```python
from build123d import *

# Parameters (mm, degrees)
SKETCH_1_R          = 48.25
EXTRUDE_1_DEPTH     = 27.7
SKETCH_2_R          = 29
EXTRUDE_2_DEPTH     = 8
SKETCH_3_R          = 29.5
SKETCH_3_R_2        = 2
SKETCH_3_R_3        = 7.5
EXTRUDE_3_DEPTH     = 6.7
SKETCH_4_R          = 1.75
CUT_EXTRUDE_1_DEPTH = 5
SKETCH_5_R          = 1.75
CUT_EXTRUDE_2_DEPTH = 5
CUT_EXTRUDE_3_DEPTH = 36.7


with BuildPart() as part:
    # 草图1 → 凸台-拉伸1 (new body)
    with BuildSketch(Plane.XY):
        Circle(SKETCH_1_R)
    extrude(amount=EXTRUDE_1_DEPTH)

    # 草图2 → 凸台-拉伸2 (add)
    with BuildSketch(Plane(origin=(0, 0, 0), x_dir=(-1, 0, 0), z_dir=(0, 0, -1))):
        Circle(SKETCH_2_R)
    extrude(amount=EXTRUDE_2_DEPTH)

    # 草图3 → 凸台-拉伸3 (add)
    with BuildSketch(Plane.XY.offset(27.7)):
        Circle(SKETCH_3_R)
        with Locations((0, 17.25)):
            Circle(SKETCH_3_R_2, mode=Mode.SUBTRACT)
        with Locations((14.938938215, 8.625)):
            Circle(SKETCH_3_R_2, mode=Mode.SUBTRACT)
        with Locations((14.938938215, -8.625)):
            Circle(SKETCH_3_R_2, mode=Mode.SUBTRACT)
        with Locations((0, -17.25)):
            Circle(SKETCH_3_R_2, mode=Mode.SUBTRACT)
        with Locations((-14.938938215, -8.625)):
            Circle(SKETCH_3_R_2, mode=Mode.SUBTRACT)
        with Locations((-14.938938215, 8.625)):
            Circle(SKETCH_3_R_2, mode=Mode.SUBTRACT)
        Circle(SKETCH_3_R_3, mode=Mode.SUBTRACT)
    extrude(amount=EXTRUDE_3_DEPTH)

    # 草图4 → 切除-拉伸1 (cut)
    with BuildSketch(Plane.XY.offset(27.7)):
        with Locations((0, 44.5)):
            Circle(SKETCH_4_R)
        with Locations((31.466251763, 31.466251763)):
            Circle(SKETCH_4_R)
        with Locations((31.466251763, -31.466251763)):
            Circle(SKETCH_4_R)
        with Locations((0, -44.5)):
            Circle(SKETCH_4_R)
        with Locations((-31.466251763, -31.466251763)):
            Circle(SKETCH_4_R)
        with Locations((-31.466251763, 31.466251763)):
            Circle(SKETCH_4_R)
        with Locations((-42.5, 0)):
            Circle(SKETCH_4_R)
        with Locations((42.5, 0)):
            Circle(SKETCH_4_R)
    extrude(amount=-CUT_EXTRUDE_1_DEPTH, mode=Mode.SUBTRACT)

    # 草图5 → 切除-拉伸2 (cut)
    with BuildSketch(Plane(origin=(0, 0, 0), x_dir=(-1, 0, 0), z_dir=(0, 0, -1))):
        with Locations((0, 42.5)):
            Circle(SKETCH_5_R)
        with Locations((30.0520382, 30.0520382)):
            Circle(SKETCH_5_R)
        with Locations((42.5, 0)):
            Circle(SKETCH_5_R)
        with Locations((30.0520382, -30.0520382)):
            Circle(SKETCH_5_R)
        with Locations((0, -42.5)):
            Circle(SKETCH_5_R)
        with Locations((-30.0520382, -30.0520382)):
            Circle(SKETCH_5_R)
        with Locations((-42.5, 0)):
            Circle(SKETCH_5_R)
        with Locations((-30.0520382, 30.0520382)):
            Circle(SKETCH_5_R)
    extrude(amount=-CUT_EXTRUDE_2_DEPTH, mode=Mode.SUBTRACT)

    # 草图6 → 切除-拉伸3 (cut, through all)
    with BuildSketch(Plane.XY.offset(27.7)):
        with BuildLine():
            Line((-46.25, 13.747727085), (-46.25, -13.747727085))
            ThreePointArc((-46.25, -13.747727085), (-48.25, 0), (-46.25, 13.747727085))
        make_face()
        with BuildLine():
            Line((46.25, -13.747727085), (46.25, 13.747727085))
            ThreePointArc((46.25, 13.747727085), (48.25, 0), (46.25, -13.747727085))
        make_face()
    extrude(amount=-CUT_EXTRUDE_3_DEPTH, mode=Mode.SUBTRACT)


solid = part.part
```
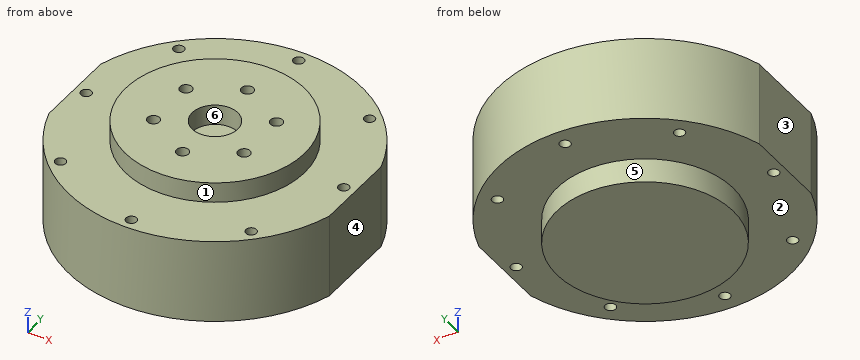
Here's how the part is built. I have some questions about the finished solid (model axes, mm). Face numbers are marked on the shaded views. A direction names the side the tool comes from. Round coordinates to 2 decimals unless told otherwise and drop trailing zeros. Loops run counter-clockwise (first coordinate to the right, second up) from the corner with the lowest first, then second, coordinate; pieces in that order, holes last.
1. Suppose I cut it at B-B, the plane x = -19.5. Please give me the cut outline in (y, z), and give its area (3 significant figures).
Answers:
outline: (-44.13, 0) - (-21.47, 0) - (-21.47, -8) - (21.47, -8) - (21.47, 0) - (44.13, 0) - (44.13, 27.7) - (22.14, 27.7) - (22.14, 34.4) - (-22.14, 34.4) - (-22.14, 27.7) - (-44.13, 27.7) - close
area: 3,090 mm2
2. For the marked faces 1, 2 and 3, which set-ups out of +Z, -Z, +X, -X, +Y, -Y let a thin tool reach every point of the face, with its end or its side?
Answers:
face 1: +Z
face 2: -Z
face 3: +Z, -Z, -X, +Y, -Y
3. Will these pins go through, and if not, where does the flat tip stop? pin 1 (1.5 mm diameter, centred on x = -19, z = 15, fed in from -Y); pin 2 (1.8 mm diameter, centred on x = -0.5, y = 42.5, fed in from -Z); pin 3 (3 mm diameter, centred on x = 31.47, y = -31.47, fed in from +Z); pin 4 (4.5 mm diameter, centred on x = -1, y = 18, fed in from +Z).
Answers:
pin 1: stops at y = -44.67
pin 2: stops at z = 5
pin 3: stops at z = 22.7
pin 4: stops at z = 34.4
4. If I drill on probe 1 along Y at (x, z) = (30, 25.5); probe 2 along Z at (x, y) = (-33, 33.5); probe 3 along X at (y, z) = (15.5, 33), over which ranges is the centre line in solid material (lowest first)?
Answers:
probe 1: y = -37.79 to -32.42, -30.51 to 30.51, 32.42 to 37.79
probe 2: z = 0 to 27.7
probe 3: x = -25.1 to -0.97, 0.97 to 25.1
5. Suppose I cut it at D-D, the plane y = 17.25. Please give me the cut outline in (x, z).
Answers:
outline: (-45.06, 0) - (-23.31, 0) - (-23.31, -8) - (23.31, -8) - (23.31, 0) - (45.06, 0) - (45.06, 27.7) - (23.93, 27.7) - (23.93, 34.4) - (2, 34.4) - (2, 27.7) - (-2, 27.7) - (-2, 34.4) - (-23.93, 34.4) - (-23.93, 27.7) - (-45.06, 27.7) - close
6. Thinking about a two-plate mould opening in X: for the marked faces 4, 5 and 6, which applies, released by +X, released by -X, zero draft, split by the parting line, or undercut?
Answers:
face 4: released by +X
face 5: split by the parting line
face 6: undercut
7. Suppose I cut it at C-C, the plane z = 15. Please give me the cut outline in (x, y).
Answers:
outline: (-46.25, -13.75) arc R48.25 ccw to (46.25, -13.75) - (46.25, 13.75) arc R48.25 ccw to (-46.25, 13.75) - close
